Can you work these out from the model? Positions are in its coordinate system, mm. Face numbers are marked on the shaded views. A direction names the side the tool comes from. Give positions to 0.01 mm unless a question says otherwise; leave off trailing zeros. Write each loop counter-clockwise with the first axis right and the second up, starting at its lowest first coordinate (ties: lowest second). Pieces come first, ordered by that corner, then holes. Notation, with made-up numbers: (11, -6) - (47, -6) arc R17 ccw to (47, 6) - close; hole circle Ø11 at (77.5, 87.5). An arc over 180 degrees is marked (long way). Return JSON: item names as keys, results as strings. Group by question number.
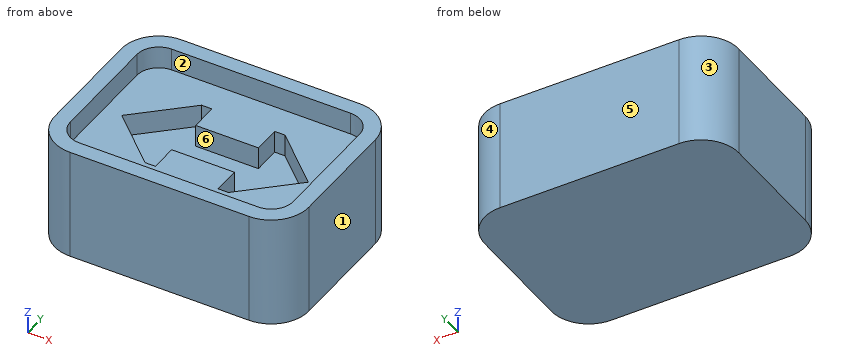
from build123d import *

# Parameters (mm, degrees)
F1_DEPTH = 5
F2_DEPTH = 4
F3_DEPTH = 3


with BuildPart() as f1:
    # F0 (on Top) → F1 (new body)
    with BuildSketch(Plane.XY):
        with BuildLine():
            Line((-4, -4.175), (4, -4.175))
            ThreePointArc((4, -4.175), (5.184404, -3.684404), (5.675, -2.5))
            Line((5.675, -2.5), (5.675, 2.5))
            ThreePointArc((5.675, 2.5), (5.184404, 3.684404), (4, 4.175))
            Line((4, 4.175), (-4, 4.175))
            ThreePointArc((-4, 4.175), (-5.184404, 3.684404), (-5.675, 2.5))
            Line((-5.675, 2.5), (-5.675, -2.5))
            ThreePointArc((-5.675, -2.5), (-5.184404, -3.684404), (-4, -4.175))
        make_face()
        with BuildLine():
            ThreePointArc((4.975, -2.5), (4.689429, -3.189429), (4, -3.475))
            Line((4, -3.475), (-4, -3.475))
            ThreePointArc((-4, -3.475), (-4.689429, -3.189429), (-4.975, -2.5))
            Line((-4.975, -2.5), (-4.975, 2.5))
            ThreePointArc((-4.975, 2.5), (-4.689429, 3.189429), (-4, 3.475))
            Line((-4, 3.475), (4, 3.475))
            ThreePointArc((4, 3.475), (4.689429, 3.189429), (4.975, 2.5))
            Line((4.975, 2.5), (4.975, -2.5))
        make_face(mode=Mode.SUBTRACT)
    extrude(amount=F1_DEPTH)

    # F0 (on Top) → F2 (join)
    with BuildSketch(Plane.XY):
        with BuildLine():
            Line((-4, -3.475), (4, -3.475))
            ThreePointArc((4, -3.475), (4.689429, -3.189429), (4.975, -2.5))
            Line((4.975, -2.5), (4.975, 2.5))
            ThreePointArc((4.975, 2.5), (4.689429, 3.189429), (4, 3.475))
            Line((4, 3.475), (-4, 3.475))
            ThreePointArc((-4, 3.475), (-4.689429, 3.189429), (-4.975, 2.5))
            Line((-4.975, 2.5), (-4.975, -2.5))
            ThreePointArc((-4.975, -2.5), (-4.689429, -3.189429), (-4, -3.475))
        make_face()
        Polygon((-1.401109, -0.899309), (-1.401059, -2.128437), (-1.864276, -2.128437), (-4.164679, 0.002819), (-1.864276, 2.128437), (-1.401059, 2.128437), (-1.401109, 0.904921), (1.401021, 0.904921), (1.401059, 2.128437), (1.864276, 2.128437), (4.164679, 0.002819), (1.864276, -2.128437), (1.401059, -2.128437), (1.40102, -0.899309), align=None, mode=Mode.SUBTRACT)
    extrude(amount=F2_DEPTH)

    # F0 (on Top) → F3 (join)
    with BuildSketch(Plane.XY):
        Polygon((-1.864276, -2.128437), (-1.401059, -2.128437), (-1.401109, -0.899309), (1.40102, -0.899309), (1.401059, -2.128437), (1.864276, -2.128437), (4.164679, 0.002819), (1.864276, 2.128437), (1.401059, 2.128437), (1.401021, 0.904921), (-1.401109, 0.904921), (-1.401059, 2.128437), (-1.864276, 2.128437), (-4.164679, 0.002819), align=None)
    extrude(amount=F3_DEPTH)


solid = f1.part
1) Will this pin go through, and if not, where does the flat tip stop? pin 1 Ø3.5 at (x, y) = (0, 0) entering from +Z.
2) I need wall thicknesses on line 1 along Y through (x, z) = (0.75, 4.3) (3 decimals); line 2 along X through (y, z) = (-2, 3.2) (3 decimals); line 3 along Y through (x, z) = (-1.5, 3.3) (3 decimals). Which ranges of each line are inside material? Lowest first, please.
3) Imagine slicing it at C-C, the plane z = 1.8. Write out the boundary of the cut face in (x, y) (3 decimals).
4) Imagine slicing it at D-D, the plane y = -3.25. Write out the boundary of the cut face in (x, z), and give its area (3 significant figures).
5) We'd pull the mould along X, two halves only. Please class the marked faces 3, 4, 5 and 6: pulls with the +X half, pulls with the -X half, needs draft (parallel to the pull), parting line crosses it, or undercut.
6) Imagine slicing it at B-B, the plane x = 0. Write out the boundary of the cut face in (y, z) (3 decimals), and give its area (3 significant figures).
7) Imagine slicing it at A-A, the plane z = 4.25. Write out the boundary of the cut face in (x, y) (3 decimals), and give its area (3 significant figures).
8) On a 3-axis mill with a long thin cutter (end or side, diameter ignored), from which of +Z, -Z, +X, -X, +Y, -Y can I reach the whole of each face in a straight line? I mean the marked faces 1 and 2. Say none if no direction works.
Resolved:
{
 "1": {"pin 1": "z = 4"},
 "2": {"line 1": "-4.175 to -3.475, 3.475 to 4.175", "line 2": "-5.675 to -2.003, -1.401 to 1.401, 2.003 to 5.675", "line 3": "-4.175 to -2.128, 2.128 to 4.175"},
 "3": {"outline": "(-5.675, -2.5) arc R1.675 ccw to (-4, -4.175) - (4, -4.175) arc R1.675 ccw to (5.675, -2.5) - (5.675, 2.5) arc R1.675 ccw to (4, 4.175) - (-4, 4.175) arc R1.675 ccw to (-5.675, 2.5) - close"},
 "4": {"outline": "(-5.5, 0) - (5.5, 0) - (5.5, 5) - (4.62, 5) - (4.62, 4) - (-4.62, 4) - (-4.62, 5) - (-5.5, 5) - close", "area": "45.7 mm^2"},
 "5": {"face 3": "pulls with the -X half", "face 4": "pulls with the +X half", "face 5": "needs draft", "face 6": "undercut"},
 "6": {"outline": "(-4.175, 0) - (4.175, 0) - (4.175, 5) - (3.475, 5) - (3.475, 4) - (0.905, 4) - (0.905, 3) - (-0.899, 3) - (-0.899, 4) - (-3.475, 4) - (-3.475, 5) - (-4.175, 5) - close", "area": "33.0 mm^2"},
 "7": {"outline": "(-5.675, -2.5) arc R1.675 ccw to (-4, -4.175) - (4, -4.175) arc R1.675 ccw to (5.675, -2.5) - (5.675, 2.5) arc R1.675 ccw to (4, 4.175) - (-4, 4.175) arc R1.675 ccw to (-5.675, 2.5) - close; hole (-4.975, -2.5) arc R0.975 ccw to (-4, -3.475) - (4, -3.475) arc R0.975 ccw to (4.975, -2.5) - (4.975, 2.5) arc R0.975 ccw to (4, 3.475) - (-4, 3.475) arc R0.975 ccw to (-4.975, 2.5) - close", "area": "24.0 mm^2"},
 "8": {"face 1": "+Z, -Z, +X, +Y, -Y", "face 2": "+Z"}
}
